Here's how the part is built. I have some questions about the finished solid (model axes, mm). A direction names the side the tool comes from. Give positions to 0.01 mm unless a question says otherwise; leave off trailing zeros. Loops run counter-clockwise (first coordinate to the right, second up) from the corner with the lowest first, then second, coordinate; pieces in that order, holes last. Notation, with made-up numbers: (-21, -24) - (4, -24) arc R21 ccw to (4, -2) - close; hole circle Ø4 at (50, 45). An arc over 180 degrees is marked (long way). Use a Markdown table: item, result.
from build123d import *

# Parameters (mm, degrees)
BOSS_EXTRUDE3_DEPTH = 10
SKETCH8_W           = 10
SKETCH8_H           = 100
CUT_EXTRUDE1_DEPTH  = 10
SKETCH9_R           = 1
CUT_EXTRUDE2_DEPTH  = 2
SKETCH11_R          = 1
CUT_EXTRUDE3_DEPTH  = 2
LPATTERN1_COUNT     = 2
LPATTERN1_PITCH     = 120


with BuildPart() as part:
    # Sketch1 → Boss-Extrude3 (new body)
    with BuildSketch(Plane(origin=(0, 0, 0), x_dir=(0, 0, -1), z_dir=(1, 0, 0))):
        with BuildLine():
            Line((7.5, 0), (14.5, 0))
            Line((14.5, 0), (14.5, 2))
            Line((14.5, 2), (9.287087811, 2))
            Line((9.287087811, 2), (9.287087811, 120))
            Line((9.287087811, 120), (14.5, 120))
            Line((14.5, 120), (14.5, 122))
            Line((14.5, 122), (9.287087811, 122))
            Line((9.287087811, 122), (-9.287087811, 122))
            Line((-9.287087811, 122), (-14.5, 122))
            Line((-14.5, 122), (-14.5, 120))
            Line((-14.5, 120), (-9.287087811, 120))
            Line((-9.287087811, 120), (-9.287087811, 2))
            Line((-9.287087811, 2), (-14.5, 2))
            Line((-14.5, 2), (-14.5, 0))
            Line((-14.5, 0), (-7.5, 0))
            ThreePointArc((-7.5, 0), (0, 7.5), (7.5, 0))
        make_face()
    extrude(amount=BOSS_EXTRUDE3_DEPTH)

    # Sketch8 → Cut-Extrude1 (cut)
    with BuildSketch(Plane(origin=(10, 0, 0), x_dir=(0, 0, -1), z_dir=(1, 0, 0))):
        with Locations((0.077954642, 63.696555082)):
            Rectangle(SKETCH8_W, SKETCH8_H)
    extrude(amount=-CUT_EXTRUDE1_DEPTH, mode=Mode.SUBTRACT)

    # Sketch9 → Cut-Extrude2 (cut)
    with BuildSketch(Plane(origin=(0, 2, 0), x_dir=(1, 0, 0), z_dir=(0, 1, 0))):
        with Locations(Location((5, 12, 0), (0, 0, 270))):
            Circle(SKETCH9_R)
    cut_extrude2 = extrude(amount=-CUT_EXTRUDE2_DEPTH, mode=Mode.SUBTRACT)

    # Sketch11 → Cut-Extrude3 (cut)
    with BuildSketch(Plane(origin=(0, 2, 0), x_dir=(1, 0, 0), z_dir=(0, 1, 0))):
        with Locations(Location((5, -12, 0), (0, 0, 270))):
            Circle(SKETCH11_R)
    cut_extrude3 = extrude(amount=-CUT_EXTRUDE3_DEPTH, mode=Mode.SUBTRACT)

    # LPattern1: Cut-Extrude2, Cut-Extrude3 ×2
    with Locations(*[(0, i * LPATTERN1_PITCH, 0) for i in range(1, LPATTERN1_COUNT)]):
        add(cut_extrude2, mode=Mode.SUBTRACT)
        add(cut_extrude3, mode=Mode.SUBTRACT)


solid = part.part
(1) Suppose I cut it at C-C on x = 7.5. Write out the boundary of the cut face in (y, z).
A:
| item | result |
|---|---|
| outline | (0, -14.5) - (2, -14.5) - (2, -9.29) - (120, -9.29) - (120, -14.5) - (122, -14.5) - (122, 14.5) - (120, 14.5) - (120, 9.29) - (2, 9.29) - (2, 14.5) - (0, 14.5) - (0, 7.5) arc R7.5 cw to (0, -7.5) - close; hole (13.7, -5.08) - (113.7, -5.08) - (113.7, 4.92) - (13.7, 4.92) - close |
(2) Suppose I cut it at A-A on z = 0. Write out the boundary of the cut face in (x, y).
A:
| item | result |
|---|---|
| outline | (0, 7.5) - (10, 7.5) - (10, 13.7) - (0, 13.7) - close; (0, 113.7) - (10, 113.7) - (10, 122) - (0, 122) - close |
(3) On a 3-axis mill with a long thin cutter (end or side, diameter ignored), from which of +Z, -Z, +X, -X, +Y, -Y can I reach the whole of each face in a straight line? I mean faces 4 (the face through (5, 62, 9.287)), 5 (the face through (5, 113.697, 0)), 6 (the face through (5, 122, 0)), 7 (the face through (3.8, 120, -11.9)). Say none if no direction works.
A:
| item | result |
|---|---|
| face 4 | +Z, +X, -X |
| face 5 | +X, -X |
| face 6 | +Z, -Z, +X, -X, +Y |
| face 7 | -Z, +X, -X |
(4) Will these pins go through, and if not, where does the flat tip stop? pin 1 (1.2 mm diameter, centred on x = 5, z = 12, fed in from +Y); pin 2 (4 mm diameter, centred on x = 6, y = 92.5, fed in from +Z); pin 3 (1 mm diameter, centred on x = 3.5, z = 1.5, fed in from -Y); pin 4 (1 mm diameter, centred on x = 2, y = 72.5, fed in from -Z).
A:
| item | result |
|---|---|
| pin 1 | through |
| pin 2 | z = 9.29 |
| pin 3 | y = 7.23 |
| pin 4 | z = -9.29 |
(5) Suppose I cut it at B-B on y = 45. Write out the boundary of the cut face in (x, z), plus the area to 3 significant figures.
A:
| item | result |
|---|---|
| outline | (0, -9.29) - (10, -9.29) - (10, -5.08) - (0, -5.08) - close; (0, 4.92) - (10, 4.92) - (10, 9.29) - (0, 9.29) - close |
| area | 85.7 mm2 |
(6) If I drill on line 1 (Z direction, x = 1.75, y = 27.5); line 2 (X direction, y = 120.8, z = -12); line 3 (Y direction, x = 2.5, z = -9.75), over which ranges is the centre line in solid material (lowest first)?
A:
| item | result |
|---|---|
| line 1 | -9.29 to -5.08, 4.92 to 9.29 |
| line 2 | 0 to 4, 6 to 10 |
| line 3 | 0 to 2, 120 to 122 |
(7) We'd pull the mould along X, two halves only. Please class faces 1 (the face through (5.676, 121.014, -12.737)), 2 (the face through (3.8, 2, -11.9)), 3 (the face through (0, 70.3, 5.4)): pulls with the +X half, pulls with the -X half, needs draft (parallel to the pull), parting line crosses it, or undercut.
A:
| item | result |
|---|---|
| face 1 | undercut |
| face 2 | needs draft |
| face 3 | pulls with the -X half |
